Autodesk Inventor part; units mm, degrees
ref_plane "YZ Plane" through (0, 0, 0) normal (1, 0, 0) x (0, 1, 0)
ref_plane "XZ Plane" through (0, 0, 0) normal (0, 1, 0) x (-1, 0, 0)
ref_plane "XY Plane" through (0, 0, 0) normal (0, 0, 1) x (1, 0, 0)
sketch "스케치1" plane through (0, 0, 0) normal (0, 0, 1) x (1, 0, 0)
  line L0 (0, 0) -> (8.4, 0)
  line L1 (8.4, 0) -> (8.4, 2.38)
  line L2 (8.4, 2.38) -> (0, 2.38)
  line L3 (0, 2.38) -> (0, 0)
  dimension "d0" = 8.4
  dimension "d1" = 2.38
extrude "돌출1" add sketch "스케치1" along normal blind 6.7
fillet "모깎기1" radius 1.19 4 edges at (8.4, 2.38, 3.35) (8.4, 0, 3.35) (0, 2.38, 3.35) (0, 0, 3.35)
sketch "스케치2" plane through (0, 0, 0) normal (0, 0, -1) x (-1, 0, 0)
  arc A0 (-7.21, 2.38) -> (-7.21, 0) centre (-7.21, 1.19) ccw
  arc A1 (-1.19, 0) -> (-1.19, 2.38) centre (-1.19, 1.19) ccw
  line L0 (-7.21, 2.38) -> (-1.19, 2.38)
  arc A2 (-7.21, 2.38) -> (-7.21, 0) centre (-7.21, 1.19) ccw
  line L1 (-1.19, 0) -> (-7.21, 0)
  arc A3 (-1.19, 0.3) -> (-1.19, 2.08) centre (-1.19, 1.19) ccw
  line L2 (-1.19, 0.3) -> (-7.21, 0.3)
  arc A4 (-7.21, 2.08) -> (-7.21, 0.3) centre (-7.21, 1.19) ccw
  line L3 (-7.21, 2.08) -> (-1.19, 2.08)
  point P0 (0, 0)
  dimension "d5" = 0.3
extrude "돌출2" cut sketch "스케치2" against normal blind 6 contours L2 A4 L3 A3
sketch "스케치3" plane through (0, 0, 6.7) normal (0, 0, 1) x (1, 0, 0)
  line L0 (7.21, 2.38) -> (1.19, 2.38)
  line L1 (4.2, 2.38) -> (4.2, 0)
  line L2 (1.19, 0) -> (7.21, 0)
  line L3 (4.2, 1.19) -> (0, 1.19)
  arc A0 (1.19, 2.38) -> (1.19, 0) centre (1.19, 1.19) ccw
  line L4 (4.2, 1.19) -> (8.4, 1.19)
  arc A1 (7.21, 0) -> (7.21, 2.38) centre (7.21, 1.19) ccw
  line L5 (-2.3, -2.01) -> (10.7, -2.01)
  line L6 (10.7, -2.01) -> (10.7, 4.39)
  line L7 (10.7, 4.39) -> (-2.3, 4.39)
  line L8 (-2.3, 4.39) -> (-2.3, -2.01)
  line L9 (-2.3, -2.01) -> (10.7, 4.39) construction
  line L10 (10.7, -2.01) -> (-2.3, 4.39) construction
  line L11 (-2.3, -2.01) -> (10.7, -2.01) construction
  point P0 (0, 0)
  dimension "d8" = 13
  dimension "d9" = 0
  dimension "d10" = 6.4
extrude "돌출3" add sketch "스케치3" along normal blind 18.8 contours A1 L4 L1 L0 | L1 L3 A0 L0 | A1 L2 L1 L4 | L1 L2 A0 L3 | L8 L7 L6 L5
fillet "모깎기2" radius 3.2 4 edges at (10.7, 4.39, 16.1) (10.7, -2.01, 16.1) (-2.3, 4.39, 16.1) (-2.3, -2.01, 16.1)
sketch "스케치4" plane through (0.9, -2.01, 6.7) normal (0, -1, 0) x (1, 0, 0)
  line L0 (0.29, 0) -> (6.31, 0)
  line L1 (3.3, 0) -> (3.3, 13.4)
  line L2 (3.3, 0) -> (16.7, 0) construction
  line L3 (9.65, 16.55) -> (-3.05, 16.55)
  line L4 (-3.05, 16.55) -> (-3.05, 10.25)
  line L5 (-3.05, 10.25) -> (9.65, 10.25)
  line L6 (9.65, 10.25) -> (9.65, 16.55)
  line L7 (9.65, 16.55) -> (-3.05, 10.25) construction
  line L8 (-3.05, 16.55) -> (9.65, 10.25) construction
  line L9 (9.65, 16.55) -> (22.35, 16.55) construction
  point P0 (-0.9, -6.7)
  dimension "d14" = 13.4
  dimension "d15" = 90
  dimension "d16" = 12.7
  dimension "d17" = 180
  dimension "d18" = 6.3
extrude "돌출4" add sketch "스케치4" along normal blind 7.4 and the other way blind 3
fillet "모깎기3" radius 3.15 4 edges at (10.55, -4.5943, 16.95) (10.55, -4.5943, 23.25) (-2.15, -4.5943, 16.95) (-2.15, -4.5943, 23.25)
sketch "스케치5" plane through (0.9, -9.41, 6.7) normal (0, -1, 0) x (1, 0, 0)
  arc A0 (0.1, 16.55) -> (0.1, 10.25) centre (0.1, 13.4) ccw
  line L0 (0.1, 10.25) -> (6.5, 10.25)
  arc A1 (6.5, 10.25) -> (6.5, 16.55) centre (6.5, 13.4) ccw
  line L1 (6.5, 16.55) -> (0.1, 16.55)
  line L2 (6.5, 11.85) -> (0.1, 11.85)
  arc A2 (0.1, 14.95) -> (0.1, 11.85) centre (0.1, 13.4) ccw
  line L3 (0.1, 14.95) -> (6.5, 14.95)
  arc A3 (6.5, 11.85) -> (6.5, 14.95) centre (6.5, 13.4) ccw
  point P0 (-0.9, -6.7)
  dimension "d24" = 1.6
extrude "돌출5" cut sketch "스케치5" against normal blind 9.6 contours L2 A2 L3 A3
properties part number "usb_connect"
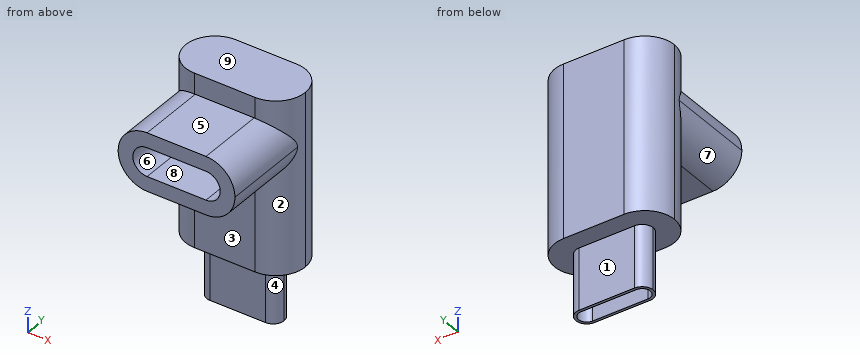
Build history of the part. All positions in model axes, mm. Face numbers are marked on the shaded views. A direction names the side the tool comes from. Coordinates: 2 decimals unless noted, no trailing zeros. Order: outer loops, then holes, each group sorted by start corner. A loop starts at its lowest first (then second) coordinate and runs counter-clockwise, first axis right, second up. Notation, with made-up numbers: (-18.5, 31.25) -> (21.5, 31.25) arc R25 ccw to (21.5, 70.25) -> close; hole circle Ø7 at (82.25, -14). An arc over 180 degrees is marked (long way). Answer in a Markdown table with one row per item. Add a question column.
Q1. Drop flat-ended pins along their axis: pin 1 (3.5 mm diameter, centred on x = 6.5, z = 20, fed in from -Y); pin 2 (3 mm diameter, centred on x = 4, z = 5, fed in from +Y); pin 3 (5 mm diameter, centred on x = 3.5, y = -6.5, fed in from +Z); pin 4 (3 mm diameter, centred on y = -3.5, z = 19.5, fed in from +X). Give the stop position or say it passes through.
Q2. Band-saw the part on D-D, the plane x = 2.5. List the corners of the cut face in (y, z).
Q3. Which spindle directions (+Z, -Z, +X, -X, +Y, -Y) get a long thin tool onto all of the face, cutting with end or side? Do the marked faces 1, 2, 3, 4 and 5. Say none if no direction does.
Q4. Wall check: line 1 along Z through (x, y) = (4.5, -5); line 2 along Z through (x, y) = (6, -1.75); line 3 along Y through (x, z) = (2.75, 7.5). Give the ranges that are in metal, low to high. Write a range as [from, to].
Q5. Mould opens along X. For the marked faces 6, 7, 8 and 9 say: +X half, -X half, draft (parallel to the pull), parting line (faces both ways), or undercut.
Answers follow:
| question | item | result |
|---|---|---|
| 1 | pin 1 | y = -9.41 |
| 1 | pin 2 | y = 2.38 |
| 1 | pin 3 | z = 23.25 |
| 1 | pin 4 | x = 10.55 |
| 2 | outline | (-9.41, 16.95) -> (-2.01, 16.95) -> (-2.01, 6.7) -> (0, 6.7) -> (0, 0) -> (0.3, 0) -> (0.3, 6) -> (2.08, 6) -> (2.08, 0) -> (2.38, 0) -> (2.38, 6.7) -> (4.39, 6.7) -> (4.39, 25.5) -> (-2.01, 25.5) -> (-2.01, 23.25) -> (-9.41, 23.25) -> (-9.41, 21.65) -> (0.19, 21.65) -> (0.19, 18.55) -> (-9.41, 18.55) -> close |
| 3 | face 1 | -Z, +X, -X, +Y |
| 3 | face 2 | +X, -Y |
| 3 | face 3 | -Z, +X, -X, -Y |
| 3 | face 4 | -Z, +X, -Y |
| 3 | face 5 | +Z, +X, -X, -Y |
| 4 | line 1 | [16.95, 18.55], [21.65, 23.25] |
| 4 | line 2 | [6.7, 18.55], [21.65, 25.5] |
| 4 | line 3 | [-2.01, 4.39] |
| 5 | face 6 | undercut |
| 5 | face 7 | -X half |
| 5 | face 8 | undercut |
| 5 | face 9 | draft |
